```python
from build123d import *

# Parameters (mm, degrees)
F1_DEPTH = 1


with BuildPart() as f1:
    # F0 (on Front) → F1 (new body)
    with BuildSketch(Plane.XZ):
        with BuildLine():
            Line((0, 120.4), (0, 0))
            Line((0, 0), (0, -120.4))
            ThreePointArc((0, -120.4), (5.857864, -134.542136), (20, -140.4))
            Line((20, -140.4), (40.775028, -140.4))
            ThreePointArc((40.775028, -140.4), (42.097903, -140.77868), (43.020022, -141.8))
            ThreePointArc((43.020022, -141.8), (46.708497, -145.885281), (52, -147.4))
            Line((52, -147.4), (80, -147.4))
            Line((80, -147.4), (80, 0))
            Line((80, 0), (80, 147.4))
            Line((80, 147.4), (52, 147.4))
            ThreePointArc((52, 147.4), (46.708497, 145.885281), (43.020022, 141.8))
            ThreePointArc((43.020022, 141.8), (42.097903, 140.77868), (40.775028, 140.4))
            Line((40.775028, 140.4), (20, 140.4))
            ThreePointArc((20, 140.4), (5.857864, 134.542136), (0, 120.4))
        make_face()
    extrude(amount=F1_DEPTH)


solid = f1.part
```
Read the model definition and answer for the solid it produces. Units are mm, in the model's axes. Coordinates: 2 decimals unless noted, no trailing zeros. Write each loop counter-clockwise with the first axis right and the second up, starting at its lowest first coordinate (ties: lowest second). Pieces come first, ordered by that corner, then holes. Notation, with made-up numbers: (70.25, 31) - (96.25, 31) arc R37 ccw to (96.25, 68) - close; hole circle Ø10 at (34.5, 78.5). An arc over 180 degrees is marked (long way). Answer as a JSON object with one key per item and string values. Group by question number.
1. A cutting plane is placed at C-C (x = 6). Determine the outline of the cut face in (y, z), plus the area to 3 significant figures.
2. A cutting plane is placed at A-A (y = -0.35). Determine the outline of the cut face in (x, z), plus the area to 3 significant figures.
3. A cutting plane is placed at B-B (x = 33.5). Determine the outline of the cut face in (y, z).
4. This flat-tipped pin is pushed along its axis until it touches: P1, Ø8, axis at x = 71.5, z = -45, coming from the +Y side. Where does it stop, or does it pass through?
5. Consider L1, parallel to Z at x = 32, y = -0.25; L2, parallel to Z at x = 5, y = -0.5; L3, parallel to X at y = -0.05, z = 129.5. Determine where each line is inside the solid, lowest interval first. Write a range as [from, to].
Worked out:
{
 "1": {"outline": "(-1, -134.68) - (0, -134.68) - (0, 134.68) - (-1, 134.68) - close", "area": "269 mm²"},
 "2": {"outline": "(0, -120.4) arc R20 ccw to (20, -140.4) - (40.78, -140.4) arc R2.5 cw to (43.02, -141.8) arc R10 ccw to (52, -147.4) - (80, -147.4) - (80, 147.4) - (52, 147.4) arc R10 ccw to (43.02, 141.8) arc R2.5 cw to (40.78, 140.4) - (20, 140.4) arc R20 ccw to (0, 120.4) - close", "area": "22,800 mm²"},
 "3": {"outline": "(-1, -140.4) - (0, -140.4) - (0, 140.4) - (-1, 140.4) - close"},
 "4": {"P1": "stops at y = 0"},
 "5": {"L1": "z = [-140.4, 140.4]", "L2": "z = [-133.63, 133.63]", "L3": "x = [2.19, 80]"}
}
